Build history of the part. All positions in model axes, mm. A direction names the side the tool comes from. Give positions to 0.01 mm unless a question says otherwise; leave off trailing zeros. Loops run counter-clockwise (first coordinate to the right, second up) from the corner with the lowest first, then second, coordinate; pieces in that order, holes last.
1) Band-saw the part on A-A on y = 0. List the corners of the cut face in (x, z), then the cut area to 3 significant figures.
2) Two-plate mould, pull along Y, no slides. Class faces 1 (the cylindrical face through (-9.85, -0.1, 16.48)), 2 (the cylindrical face through (8.15, 0.08, 16.48)), 3 (the flat face through (9, 0, 18)): +Y half, -Y half, draft (parallel to the pull), parting line (faces both ways), or undercut.
3) Wall check: line 1 (Y direction, x = 0, z = 3.25); line 2 (X direction, y = 3.5, z = 14.25); line 3 (X direction, y = 3, z = 17.75). Give the ranges that are in metal, low to high.
4) Flat gauge pins, fed straight in: P1, Ø6, axis at x = 7.5, z = 9, coming from the -Y side; P2, Ø11.5, axis at x = 0, y = 0, coming from the +Z side; P3, Ø4, axis at y = 6, z = 9.5, coming from the -X side. Where does each tip first touch, or does it go through?
5) Band-saw the part on C-C on z = 4. List the corners of the cut face in (x, y), then the cut area to 3 significant figures.
6) 3-axis set-ups, long thin cutter, end or side, ignore diameter. For faces 4 (the flat face through (-4.358, 7.861, 16.479)), 5 (the flat face through (-7.78, -4.49, 16.48)), 6 (the cylindrical face through (9.85, 0.1, 16.48)), 7 (the cylindrical face through (-8.15, -0.08, 16.48)): which of +Z, -Z, +X, -X, +Y, -Y reach the whole face in a straight line?
```python
from build123d import *

# Parameters (mm, degrees)
SKETCH_R     = 10
SKETCH_R_2   = 5
PAD_DEPTH    = 15
PAD001_DEPTH = 3
FILLET_R     = 3


with BuildPart() as part:
    # Sketch → Pad (new body)
    with BuildSketch(Plane.XY):
        Circle(SKETCH_R)
        Circle(SKETCH_R_2, mode=Mode.SUBTRACT)
    extrude(amount=PAD_DEPTH)

    # Sketch001 (on Face4 of Pad) → Pad001 (join)
    with BuildSketch(Plane.XY.offset(15)):
        with BuildLine():
            ThreePointArc((-8.697034, 4.624295), (-9.8485, -0.171906), (-8.53035, -4.925))
            Line((-7.058107, -4.075), (-8.53035, -4.925))
            ThreePointArc((-7.196023, 3.826193), (-8.148759, -0.142237), (-7.058107, -4.075))
            Line((-7.196023, 3.826193), (-8.697034, 4.624295))
        make_face()
        with BuildLine():
            Line((-3.951198, 7.128151), (-4.775375, 8.615004))
            ThreePointArc((4.775375, 8.615004), (0, 9.85), (-4.775375, 8.615004))
            Line((3.951198, 7.128151), (4.775375, 8.615004))
            ThreePointArc((3.951198, 7.128151), (0, 8.15), (-3.951198, 7.128151))
        make_face()
        with BuildLine():
            Line((3.951198, -7.128151), (4.775375, -8.615004))
            ThreePointArc((-4.775375, -8.615004), (0, -9.85), (4.775375, -8.615004))
            Line((-3.951198, -7.128151), (-4.775375, -8.615004))
            ThreePointArc((-3.951198, -7.128151), (0, -8.15), (3.951198, -7.128151))
        make_face()
        with BuildLine():
            Line((7.058107, 4.075), (8.53035, 4.925))
            ThreePointArc((8.697034, -4.624295), (9.8485, 0.171906), (8.53035, 4.925))
            Line((7.196023, -3.826193), (8.697034, -4.624295))
            ThreePointArc((7.196023, -3.826193), (8.148759, 0.142237), (7.058107, 4.075))
        make_face()
    extrude(amount=PAD001_DEPTH)

    # Fillet
    fillet_edges = [part.edges().sort_by_distance(p)[0] for p in [
        (-10, 0, 0),
    ]]
    fillet(fillet_edges, radius=FILLET_R)


solid = part.part
```
Findings below:
1. outline: (-10, 3) arc R3 ccw to (-7, 0) - (-5, 0) - (-5, 15) - (-8.15, 15) - (-8.15, 18) - (-9.85, 18) - (-9.85, 15) - (-10, 15) - close; (5, 0) - (7, 0) arc R3 ccw to (10, 3) - (10, 15) - (9.85, 15) - (9.85, 18) - (8.15, 18) - (8.15, 15) - (5, 15) - close
1. area: 156 mm2
2. face 1: parting line
2. face 2: undercut
2. face 3: draft
3. line 1: y = -10 to -5, 5 to 10
3. line 2: x = -9.37 to -3.57, 3.57 to 9.37
3. line 3: x = -9.38 to -7.58, 7.58 to 9.38
4. P1: stops at y = -8.93
4. P2: stops at z = 15
4. P3: stops at x = -9.17
5. outline: circle Ø20 at (0, 0); hole circle Ø10 at (0, 0)
5. area: 236 mm2
6. face 4: +Z, -X
6. face 5: +Z, -Y
6. face 6: +Z, +X
6. face 7: +Z
